The listing builds one solid part. Answer for the finished solid, in the listing's coordinates (mm). Give positions to 0.01 mm unless a question says otherwise; leave off trailing zeros. Loops run counter-clockwise (first coordinate to the right, second up) from the corner with the lowest first, then second, coordinate; pieces in that order, holes last.
Item 1: Section A-A, the plane z = 1.25 is taken. Give the vertices of the cut face in (x, y) (3 decimals).
Item 2: Section D-D, the plane z = -3.5 is taken. Give the vertices of the cut face in (x, y) (3 decimals), and give its area (3 significant figures).
Item 3: Consider line 1 along X through (y, z) = (-1.4, 1) (3 decimals); line 2 along X through (y, z) = (-4.25, 1.75) (3 decimals); line 3 along Z through (x, y) = (-18, -4.1). Determine where each line is inside the solid, lowest interval first.
Item 4: Section C-C, the plane x = -19 is taken. Give the vertices of the cut face in (y, z), and give its area (3 significant figures).
Item 5: The mould has two halves that part along X. Classify faces 1 (the face through (-14, -3, 4.762)), 2 (the face through (15.989, -2.504, 2.348)), 3 (the face through (22.413, -2.504, 2.415)), 4 (the face through (-41.275, -3, 2)): pulls with the +X half, pulls with the -X half, needs draft (parallel to the pull), parting line crosses it, or undercut.
from build123d import *

# Parameters (mm, degrees)
F1_DEPTH = 5.08


with BuildPart() as f1:
    # F0 (on Front) → F1 (new body)
    with BuildSketch(Plane.XZ):
        Polygon((-16.462963, -4.7625), (41.275, -4.7625), (41.275, 0), (19.05, 0), (12.84111, 4.7625), (-41.275, 4.7625), (-41.275, 0), align=None)
        Polygon((19.05, 0), (41.275, 0), (41.275, 4.7625), (25.682222, 4.7625), align=None)
    extrude(amount=F1_DEPTH)


solid = f1.part
Worked answers:
1. outline: (-41.275, -5.08) - (17.42, -5.08) - (17.42, 0) - (-41.275, 0) - close; (20.791, -5.08) - (41.275, -5.08) - (41.275, 0) - (20.791, 0) - close
2. outline: (-23.04, -5.08) - (41.275, -5.08) - (41.275, 0) - (-23.04, 0) - close
2. area: 327 mm2
3. line 1: x = -41.275 to 17.746, 20.443 to 41.275
3. line 2: x = -41.275 to 16.769, 21.487 to 41.275
3. line 3: z = -4.47 to 4.76
4. outline: (-5.08, -4.28) - (0, -4.28) - (0, 4.76) - (-5.08, 4.76) - close
4. area: 45.9 mm2
5. face 1: needs draft
5. face 2: undercut
5. face 3: undercut
5. face 4: pulls with the -X half
